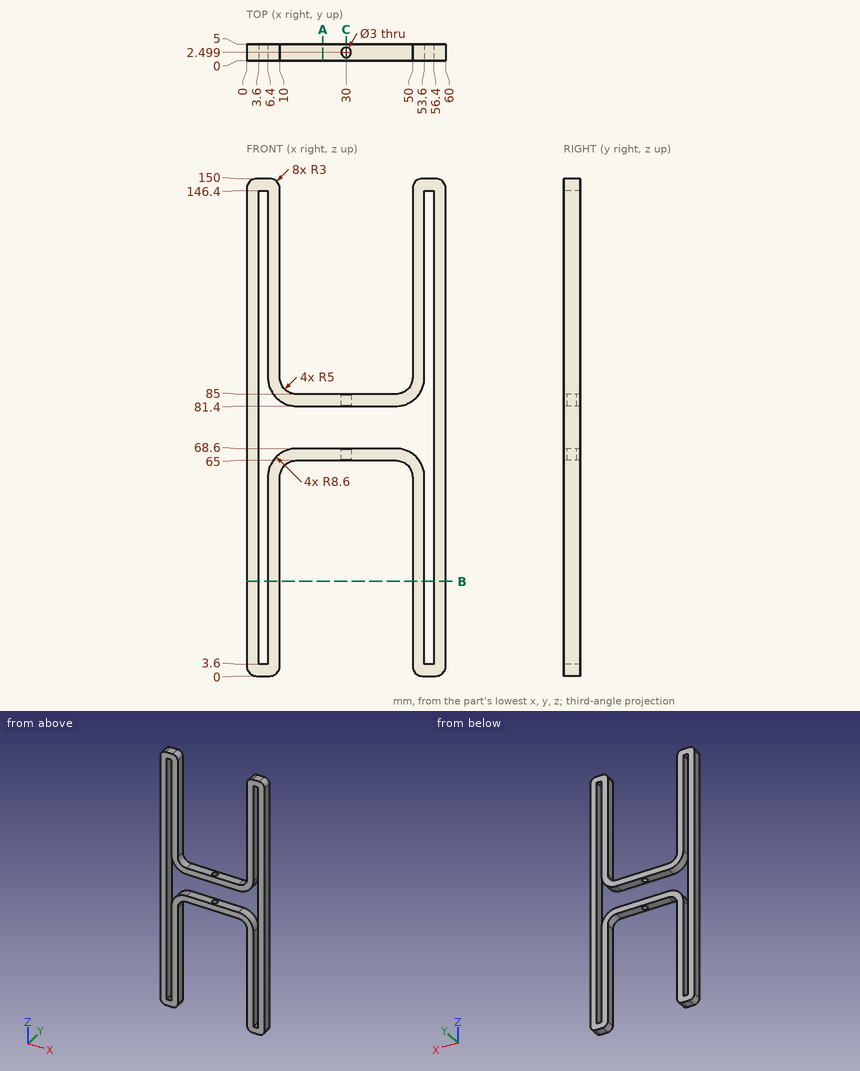
Study the drawing (mm; zero at the part's minimum x, y, z) and answer. Coordinates: 2 decimals unless noted, no trailing zeros. Write each loop counter-clockwise with the first axis right and the second up, starting at its lowest first coordinate (ties: lowest second). Pieces come first, ordered by that corner, then holes. Notation, with made-up numbers: (36.5, 35.25) - (61.5, 35.25) arc R30 ccw to (61.5, 64.25) - close; hole circle Ø10 at (51, 27). An arc over 180 degrees is marked (long way). Return JSON: item names as keys, results as strings. Group by question number.
1. A cutting plane is placed at A-A, the plane x = 23. Determine the outline of the cut face in (y, z), plus the area to 3 significant figures.
2. A cutting plane is placed at C-C, the plane x = 30. Determine the outline of the cut face in (y, z), plus the area to 3 significant figures.
3. Given pin 1 (1.5 mm diameter, centred on x = 34, y = 3.5, fed in from -Z), flat-ended and moving along its own axis, determine where the tip first touches the part or whether it passes through.
4. Straight lines are drawn through the part: L1, parallel to X at y = 4.45, z = 38; L2, parallel to Z at x = 38, y = 2.15; L3, parallel to Y at x = 30, z = 82.7. For each, find the intervals that lie inside material, in ascending order.
5. A cutting plane is placed at B-B, the plane z = 28.5. Determine the outline of the cut face in (x, y), plus the area to 3 significant figures.
Ans:
{
 "1": {"outline": "(0, 65) - (5, 65) - (5, 68.6) - (0, 68.6) - close; (0, 81.4) - (5, 81.4) - (5, 85) - (0, 85) - close", "area": "36.0 mm²"},
 "2": {"outline": "(0, 65) - (1, 65) - (1, 68.6) - (0, 68.6) - close; (0, 81.4) - (1, 81.4) - (1, 85) - (0, 85) - close; (4, 65) - (5, 65) - (5, 68.6) - (4, 68.6) - close; (4, 81.4) - (5, 81.4) - (5, 85) - (4, 85) - close", "area": "14.4 mm²"},
 "3": {"pin 1": "z = 65"},
 "4": {"L1": "0 to 3.6, 6.4 to 10, 50 to 53.6, 56.4 to 60", "L2": "65 to 68.6, 81.4 to 85", "L3": "0 to 1, 4 to 5"},
 "5": {"outline": "(0, 0) - (3.6, 0) - (3.6, 5) - (0, 5) - close; (6.4, 0) - (10, 0) - (10, 5) - (6.4, 5) - close; (50, 0) - (53.6, 0) - (53.6, 5) - (50, 5) - close; (56.4, 0) - (60, 0) - (60, 5) - (56.4, 5) - close", "area": "72.0 mm²"}
}
